from build123d import *

# Parameters (mm, degrees)
SKETCH1_R           = 4.95
SKETCH1_R_2         = 4.15
BOSS_EXTRUDE1_DEPTH = 10
CHAMFER1_SIZE       = 0.2
SKETCH2_R           = 2.1
CUT_EXTRUDE1_DEPTH  = 13.206760422


with BuildPart() as part:
    # Sketch1 → Boss-Extrude1 (new body)
    with BuildSketch(Plane.XY):
        Circle(SKETCH1_R)
        Circle(SKETCH1_R_2, mode=Mode.SUBTRACT)
    extrude(amount=BOSS_EXTRUDE1_DEPTH)

    # Chamfer1
    chamfer1_edges = [part.edges().sort_by_distance(p)[0] for p in [
        (-4.95, 0, 0),
        (-4.15, 0, 0),
        (-4.15, 0, 10),
    ]]
    chamfer(chamfer1_edges, length=CHAMFER1_SIZE)

    # Sketch2 → Cut-Extrude1 (cut, through all)
    with BuildSketch(Plane(origin=(0, 0, 0), x_dir=(1, 0, 0), z_dir=(0, 1, 0))):
        with Locations(Location((0, -3.9, 0), (0, 0, 270))):
            Circle(SKETCH2_R)
    extrude(amount=-CUT_EXTRUDE1_DEPTH, mode=Mode.SUBTRACT)


solid = part.part
Read the model definition and answer for the solid it produces. Units are mm, in the model's axes. Give positions to 0.01 mm unless a question says otherwise; leave off trailing zeros. Write each loop counter-clockwise with the first axis right and the second up, starting at its lowest first coordinate (ties: lowest second). Pieces come first, ordered by that corner, then holes. Notation, with made-up numbers: (-39.5, 81.25) - (-33.5, 81.25) arc R32 ccw to (-33.5, 107.25) - close; hole circle Ø7 at (82.5, -4). An arc over 180 degrees is marked (long way). Answer in a Markdown table with one row per item. Add a question column.
Item 1: Section A-A, the plane x = 0 is taken. Write down the section's boundary in (y, z), and give its area (3 significant figures).
Item 2: Section D-D, the plane z = 3.9 is taken. Write down the section's boundary in (x, y), and give its area (3 significant figures).
Item 3: Section B-B, the plane y = 0 is taken. Write down the section's boundary in (x, z), and give its area (3 significant figures).
Item 4: Flat-ended cylindrical pins translate along their axes: P1, Ø1.5, axis at y = -2, z = 2, coming from the +X side; P2, Ø1.5, axis at x = -1.5, z = 2, coming from the -Y side. Find the tip coordinate at first contact, or state that the pin passes through.
Item 5: Determine the mould class of faces 1 (the face through (-0.54, 4.115, 4.933)), 2 (the face through (0.631, -4.257, 5.903)), 3 (the face through (2.661, 4.174, 5.031)) for opening direction X: pulls with the +X half, pulls with the -X half, needs draft (parallel to the pull), parting line crosses it, or undercut.
Item 6: Section C-C, the plane z = 6.5 is taken. Write down the section's boundary in (x, y).
Item 7: Find the intervals of material crossed by L1, parallel to X at y = -0.5, z = 4.75; L2, parallel to Y at x = 1, z = 1; L3, parallel to Y at x = 2, z = 4.75, in increasing order.
Recorded:
| question | item | result |
|---|---|---|
| 1 | outline | (-4.95, 0.2) - (-4.75, 0) - (-4.35, 0) - (-4.15, 0.2) - (-4.15, 1.8) - (-4.95, 1.8) - close; (-4.95, 6) - (-4.15, 6) - (-4.15, 9.8) - (-4.35, 10) - (-4.95, 10) - close; (4.15, 0.2) - (4.35, 0) - (4.75, 0) - (4.95, 0.2) - (4.95, 10) - (4.35, 10) - (4.15, 9.8) - close |
| 1 | area | 12.5 mm2 |
| 2 | outline | (-2.1, -4.48) - (-2.1, -3.58) arc R4.15 cw (long way) to (2.1, -3.58) - (2.1, -4.48) arc R4.95 ccw (long way) to start |
| 2 | area | 19.4 mm2 |
| 3 | outline | (-4.95, 0.2) - (-4.75, 0) - (-4.35, 0) - (-4.15, 0.2) - (-4.15, 9.8) - (-4.35, 10) - (-4.95, 10) - close; (4.15, 0.2) - (4.35, 0) - (4.75, 0) - (4.95, 0.2) - (4.95, 10) - (4.35, 10) - (4.15, 9.8) - close |
| 3 | area | 15.9 mm2 |
| 4 | P1 | stops at x = 4.79 |
| 4 | P2 | stops at y = -4.89 |
| 5 | face 1 | undercut |
| 5 | face 2 | undercut |
| 5 | face 3 | parting line crosses it |
| 6 | outline | circle Ø9.9 at (0, 0); hole circle Ø8.3 at (0, 0) |
| 7 | L1 | x = -4.92 to -4.12, 4.12 to 4.92 |
| 7 | L2 | y = -4.85 to -4.03, 4.03 to 4.85 |
| 7 | L3 | y = -4.53 to -3.64, 3.64 to 4.53 |
